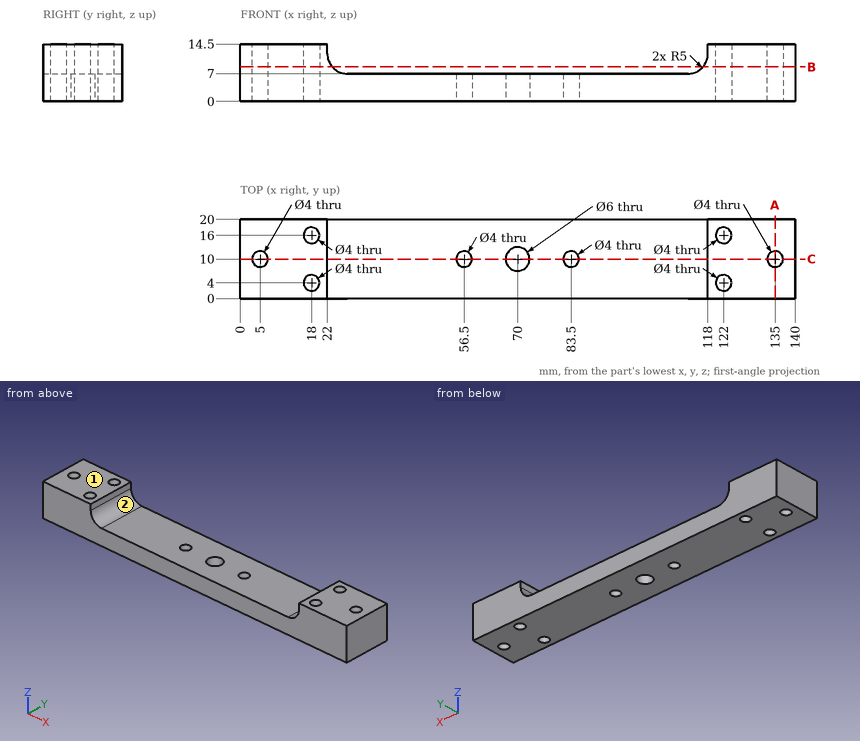
Input: dimensioned drawing with shaded views. Units: mm. Origin: part minimum x, y, z. A direction names the side the tool comes from. Round coordinates to 2 decimals unless told otherwise and drop trailing zeros. Loops run counter-clockwise (first coordinate to the right, second up) from the corner with the lowest first, then second, coordinate; pieces in that order, holes last. Notation, with made-up numbers: M 52.25,57 L 72.25,57 A23 ccw 72.25,83 Z; hole C 44.25,-37 d7. An arc over 180 degrees is marked long. Return JSON: item names as keys, results as strings. Group by question number.
1. Section query A-A on x = 135. Output: boundary loops of the cut face in (y, z).
2. Section query B-B on z = 8.75. Output: boundary loops of the cut face in (x, y).
3. Material intervals for line 1 along Y through (x, z) = (122, 9); line 2 along Y through (x, z) = (135, 11); line 3 along X through (y, z) = (5.25, 4.5), sorted ascending. Write a range as from..to.
4. Pin query (flat end, axial travel): pin 1 (8 mm diameter, centred on x = 70, y = 10, fed in from +Z). Return the tip coordinate at first contact, or that it passes through.
5. Reachability of the marked faces 1 and 2 from +Z, -Z, +X, -X, +Y, -Y: full face, straight path, thin tool, end or side. Return the list, or none.
6. Section query C-C on y = 10. State how many separate pieces and enclosed holes the cut face has, and give its area (3 significant figures).
Checks:
{
 "1": {"outline": "M 0,0 L 8,0 L 8,14.5 L 0,14.5 Z; M 12,0 L 20,0 L 20,14.5 L 12,14.5 Z"},
 "2": {"outline": "M 0,0 L 23.2,0 L 23.2,20 L 0,20 Z; M 116.8,0 L 140,0 L 140,20 L 116.8,20 Z; hole C 5,10 d4; hole C 18,4 d4; hole C 18,16 d4; hole C 122,4 d4; hole C 122,16 d4; hole C 135,10 d4"},
 "3": {"line 1": "y = 0..2, 6..14, 18..20", "line 2": "y = 0..8, 12..20", "line 3": "x = 0..16.44, 19.56..120.44, 123.56..140"},
 "4": {"pin 1": "stops at z = 7"},
 "5": {"face 1": "+Z, +X, -X, +Y, -Y", "face 2": "+Z, +Y, -Y"},
 "6": {"separate pieces": "6", "enclosed holes": "0", "area": "1,110 mm²"}
}
